The listing builds one solid part. Answer for the finished solid, in the listing's coordinates (mm). A direction names the side the tool comes from. Give positions to 0.01 mm unless a question says otherwise; leave off trailing zeros. Order: outer loops, then holes, each group sorted by start corner. A loop starts at its lowest first (then second) coordinate and runs counter-clockwise, first axis right, second up. Notation, with made-up numbers: M 12,42.5 L 59,42.5 A26 cw 59,61.5 Z; hole C -12,1 d11. An arc over 180 degrees is marked long. Answer as a JSON object with one key per item and string values. Group by question number.
```python
from build123d import *

# Parameters (mm, degrees)
SKETCH6_OUTSIDE_W       = 110.342
SKETCH6_OUTSIDE_H       = 110.342
SKETCH6_OUTSIDE_W_2     = 21
SKETCH6_OUTSIDE_H_2     = 30
CUT_EXTRUDE3_DEPTH      = 40
SKETCH4_W               = 17.5
SKETCH4_H               = 5
FILLET1_R               = 1
SKETCH8_R               = 2.5
CUT_EXTRUDE4_DEPTH      = 10.5
CUT_EXTRUDE4_DEPTH_BACK = 31.5


with BuildPart() as part:
    # Sketch1 → Revolve1 (revolve)
    with BuildSketch(Plane.XY):
        with BuildLine():
            Line((297, 15), (300, 15))
            Line((300, 15), (300, 20))
            Line((300, 20), (0, 20))
            Line((0, 20), (0, 10))
            Line((0, 10), (-18.366750419, 10))
            ThreePointArc((-18.366750419, 10), (-30.674548662, 10.573528147), (-37, 0))
            Line((-37, 0), (0, 0))
            Line((0, 0), (3, 0))
            Line((3, 0), (3, 17))
            Line((3, 17), (297, 17))
            Line((297, 17), (297, 15))
        make_face()
    revolve(axis=Axis((0, 0, 0), (1, 0, 0)))

    # Sketch6 outside → Cut-Extrude3 (cut)
    with BuildSketch(Plane.ZY):
        Rectangle(SKETCH6_OUTSIDE_W, SKETCH6_OUTSIDE_H)
        Rectangle(SKETCH6_OUTSIDE_W_2, SKETCH6_OUTSIDE_H_2, mode=Mode.SUBTRACT)
    extrude(amount=CUT_EXTRUDE3_DEPTH, mode=Mode.SUBTRACT)

    # Sketch4 → Cut-Revolve1 (revolve, cut)
    with BuildSketch(Plane(origin=(0, 0, 0), x_dir=(1, 0, 0), z_dir=(0, 1, 0))):
        with Locations((-28.25, 0)):
            Rectangle(SKETCH4_W, SKETCH4_H)
    revolve(axis=Axis((-37, 0, -2.5), (0, 0, 1)), mode=Mode.SUBTRACT)

    # Fillet1
    fillet1_edges = [part.edges().sort_by_distance(p)[0] for p in [
        (300, -20, 0),
        (0, -10, 0),
        (0, -20, 0),
    ]]
    fillet(fillet1_edges, radius=FILLET1_R)

    # Sketch8 → Cut-Extrude4 (cut, two sides)
    with BuildSketch(Plane.XY.offset(10.5)) as cut_extrude4_sk:
        with Locations((-25, 0)):
            Circle(SKETCH8_R)
    extrude(amount=CUT_EXTRUDE4_DEPTH, mode=Mode.SUBTRACT)
    extrude(cut_extrude4_sk.sketch, amount=-CUT_EXTRUDE4_DEPTH_BACK, mode=Mode.SUBTRACT)


solid = part.part
```
Item 1: A tool of negligible diameter and unlimited length cuts with its end or side. For faces 1 (the flat face through (-28, 0, -2.5)), 2 (the flat face through (-28, 0, -10.5)), 3 (the cylindrical face through (152.058, 9.139, 14.334)), 4 (the cylindrical face through (298.521, -14.985, 0.66)), from which of +Z, -Z, +X, -X, +Y, -Y can it reach the whole face along a straight path? Write none if from no direction.
Item 2: Section A-A (x = 203) is taken. Determine the outline of the cut face in (y, z).
Item 3: Consider probe 1 along Z at (x, y) = (146, -1.5); probe 2 along X at (y, z) = (16.5, -3); probe 3 along Z at (x, y) = (299, 0). Determine where each line is inside the solid, lowest interval first. Write a range as from..to.
Item 4: Determine the mould class of faces 5 (the cylindrical face through (147.914, -4.336, -19.524)), 6 (the flat face through (300, -14, 6)), 7 (the cylindrical face through (-9.8, -2.17, -9.76)) for opening direction X: released by +X, released by -X, zero draft, split by the parting line, or undercut.
Item 5: Flat-ended cylindrical pins translate along their axes: P1, Ø5, axis at x = -24, y = 2.5, coming from the +Z side; P2, Ø8, axis at x = -25, y = 0, coming from the -Z side; P3, Ø4, axis at x = 225.5, y = 4.5, coming from the +Z side; P4, Ø17, axis at y = -5.5, z = -4.5, coming from the -X side. Find the tip coordinate at first contact, or state that the pin passes through.
Values found:
{
 "1": {"face 1": "-X", "face 2": "-Z, -X, +Y, -Y", "face 3": "none", "face 4": "+X"},
 "2": {"outline": "C 0,0 d40; hole C 0,0 d34"},
 "3": {"probe 1": "z = -19.94..-16.93, 16.93..19.94", "probe 2": "x = 0..3, 297..300", "probe 3": "z = -20..-15, 15..20"},
 "4": {"face 5": "zero draft", "face 6": "released by +X", "face 7": "undercut"},
 "5": {"P1": "stops at z = 10.5", "P2": "stops at z = -10.5", "P3": "stops at z = 19.84", "P4": "stops at x = -36.74"}
}
